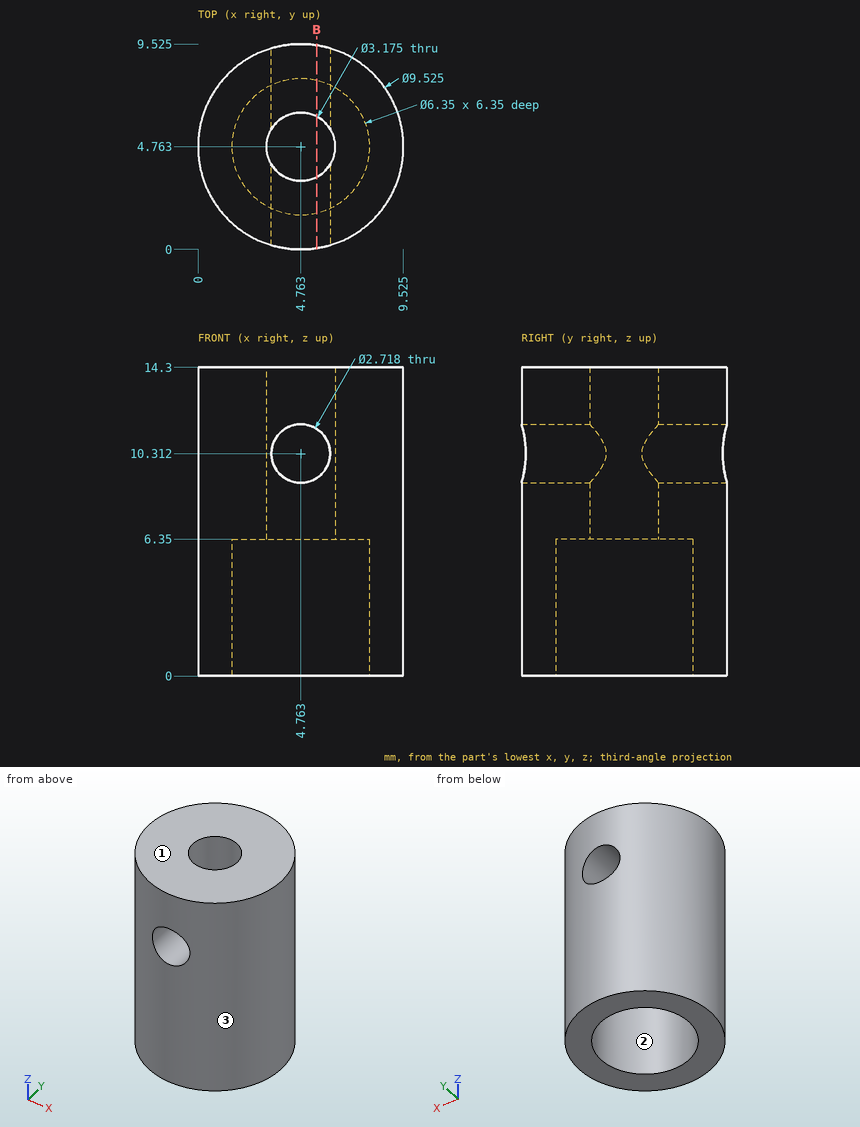
Study the drawing (mm; zero at the part's minimum x, y, z) and answer. Give positions to 0.01 mm unless a question says otherwise; leave off trailing zeros. Answer as a JSON object with one key per item and string values. Group by question number.
1) The mould has two halves that part along Y. Classify the marked faces 1, 2 and 3: +Y half, -Y half, draft (parallel to the pull), parting line (faces both ways), or undercut.
2) Find section B-B (x = 5.5). Count the separate pieces of the cut face and the enclosed holes in it.
3) Each of these flat-tipped pins is pushed along its axis until it touches: P1, Ø4.5, axis at x = 4.76, z = 10.31, coming from the -Y side; P2, Ø1.5, axis at x = 4.5, y = 7, coming from the -Z side; P3, Ø2, axis at y = 1.5, z = 9.5, coming from the -X side; P4, Ø1, axis at y = 7, z = 4, coming from the +X side. Where does it stop, or does it pass through?
4) Consider L1, parallel to Z at x = 4.5, y = 0.5 (1 decimal); L2, parallel to Y at x = 5.75, z = 7.5 (1 decimal); L3, parallel to Z at x = 6.25, y = 6. Determine where each line is inside the solid, lowest interval first. Write a range as from..to.
Values follow:
{
 "1": {"face 1": "draft", "face 2": "undercut", "face 3": "parting line"},
 "2": {"separate pieces": "4", "enclosed holes": "0"},
 "3": {"P1": "stops at y = 0", "P2": "stops at z = 6.35", "P3": "stops at x = 0.57", "P4": "stops at x = 9.2"},
 "4": {"L1": "z = 0..9, 11.6..14.3", "L2": "y = 0.1..3.5, 6..9.4", "L3": "z = 6.35..14.3"}
}
